Here's how the part is built. I have some questions about the finished solid (model axes, mm). A direction names the side the tool comes from. Round coordinates to 2 decimals unless told otherwise and drop trailing zeros. Write each loop counter-clockwise with the first axis right and the second up, starting at its lowest first coordinate (ties: lowest second). Pieces come first, ordered by that corner, then holes. Notation, with made-up numbers: (1.25, 41) -> (18.25, 41) arc R30 ccw to (18.25, 78) -> close; hole circle Ø10 at (-6.75, -20). An arc over 180 degrees is marked (long way). Answer as CSV lines item,"result".
from build123d import *

# Parameters (mm, degrees)
CROQUIS1_W              = 75
CROQUIS1_H              = 75
SALIENTE_EXTRUIR1_DEPTH = 15
REDONDEO1_R             = 8
CROQUIS2_R              = 4
CORTAR_EXTRUIR1_DEPTH   = 15
SALIENTE_EXTRUIR2_DEPTH = 30
REDONDEO2_R             = 6
CROQUIS5_R              = 3
CORTAR_EXTRUIR2_DEPTH   = 54.5
CROQUIS6_R              = 5
CORTAR_EXTRUIR4_DEPTH   = 30
CROQUIS4_R              = 23
SALIENTE_EXTRUIR4_DEPTH = 5
CROQUIS8_R              = 12.5
CORTAR_EXTRUIR6_DEPTH   = 51


with BuildPart() as part:
    # Croquis1 → Saliente-Extruir1 (new body)
    with BuildSketch(Plane(origin=(0, 0, 0), x_dir=(1, 0, 0), z_dir=(0, 1, 0))):
        Rectangle(CROQUIS1_W, CROQUIS1_H)
    extrude(amount=SALIENTE_EXTRUIR1_DEPTH)

    # Redondeo1
    redondeo1_edges = [part.edges().sort_by_distance(p)[0] for p in [
        (37.5, 7.5, 37.5),
        (-37.5, 7.5, 37.5),
        (-37.5, 7.5, -37.5),
        (37.5, 7.5, -37.5),
    ]]
    fillet(redondeo1_edges, radius=REDONDEO1_R)

    # Croquis2 → Cortar-Extruir1 (cut)
    with BuildSketch(Plane(origin=(0, 15, 0), x_dir=(1, 0, 0), z_dir=(0, 1, 0))):
        with Locations((-29.5, 29.5)):
            Circle(CROQUIS2_R)
        with Locations((-29.5, -29.5)):
            Circle(CROQUIS2_R)
        with Locations((29.5, 29.5)):
            Circle(CROQUIS2_R)
        with Locations((29.5, -29.5)):
            Circle(CROQUIS2_R)
    extrude(amount=-CORTAR_EXTRUIR1_DEPTH, mode=Mode.SUBTRACT)

    # Croquis3 → Saliente-Extruir2 (add)
    with BuildSketch(Plane(origin=(0, 15, 0), x_dir=(1, 0, 0), z_dir=(0, 1, 0))):
        with BuildLine():
            Line((-16, -28.5), (-9, -28.5))
            Line((-9, -28.5), (-9, -17.5))
            Line((-9, -17.5), (9, -17.5))
            Line((9, -17.5), (9, -28.5))
            Line((9, -28.5), (16, -28.5))
            Line((16, -28.5), (16, -12.953381025))
            Line((16, -12.953381025), (27.733418669, -9.619169527))
            ThreePointArc((27.733418669, -9.619169527), (35, 0), (27.733418669, 9.619169527))
            Line((27.733418669, 9.619169527), (16, 12.953381025))
            Line((16, 12.953381025), (16, 28.5))
            Line((16, 28.5), (9, 28.5))
            Line((9, 28.5), (9, 17.5))
            Line((9, 17.5), (-9, 17.5))
            Line((-9, 17.5), (-9, 28.5))
            Line((-9, 28.5), (-16, 28.5))
            Line((-16, 28.5), (-16, 12.953381025))
            Line((-16, 12.953381025), (-27.733418669, 9.619169527))
            ThreePointArc((-27.733418669, 9.619169527), (-35, 0), (-27.733418669, -9.619169527))
            Line((-27.733418669, -9.619169527), (-16, -12.953381025))
            Line((-16, -12.953381025), (-16, -28.5))
        make_face()
    extrude(amount=SALIENTE_EXTRUIR2_DEPTH)

    # Redondeo2
    redondeo2_edges = [part.edges().sort_by_distance(p)[0] for p in [
        (-12.5, 45, 28.5),
        (12.5, 45, 28.5),
        (12.5, 45, -28.5),
        (-12.5, 45, -28.5),
    ]]
    fillet(redondeo2_edges, radius=REDONDEO2_R)

    # Croquis5 → Cortar-Extruir2 (cut, through all)
    with BuildSketch(Plane(origin=(16, 0, 0), x_dir=(0, 0, -1), z_dir=(1, 0, 0))):
        with Locations((-22.5, 39)):
            Circle(CROQUIS5_R)
        with Locations((22.5, 39)):
            Circle(CROQUIS5_R)
    extrude(amount=-CORTAR_EXTRUIR2_DEPTH, mode=Mode.SUBTRACT)

    # Croquis6 → Cortar-Extruir4 (cut)
    with BuildSketch(Plane(origin=(0, 45, 0), x_dir=(1, 0, 0), z_dir=(0, 1, 0))):
        with Locations((-25, 0)):
            Circle(CROQUIS6_R)
        with Locations((25, 0)):
            Circle(CROQUIS6_R)
    extrude(amount=-CORTAR_EXTRUIR4_DEPTH, mode=Mode.SUBTRACT)

    # Croquis4 → Saliente-Extruir4 (add)
    with BuildSketch(Plane(origin=(0, 0, 0), x_dir=(-1, 0, 0), z_dir=(0, -1, 0))):
        Circle(CROQUIS4_R)
    extrude(amount=SALIENTE_EXTRUIR4_DEPTH)

    # Croquis8 → Cortar-Extruir6 (cut, through all)
    with BuildSketch(Plane(origin=(0, 45, 0), x_dir=(1, 0, 0), z_dir=(0, 1, 0))):
        Circle(CROQUIS8_R)
    extrude(amount=-CORTAR_EXTRUIR6_DEPTH, mode=Mode.SUBTRACT)


solid = part.part
Item 1: Will these pins go through, and if not, where does the flat tip stop? pin 1 (3.5 mm diameter, centred on x = -13, y = 29, fed in from -Z); pin 2 (5 mm diameter, centred on x = 25.5, z = 1.5, fed in from +Y); pin 3 (13 mm diameter, centred on x = -29.5, z = 29.5, fed in from -Y); pin 4 (22.5 mm diameter, centred on x = 3.5, z = -4, fed in from +Y).
Results found:
pin 1,"stops at z = -28.5"
pin 2,"stops at y = 15"
pin 3,"stops at y = 0"
pin 4,"stops at y = 45"
Item 2: Suppose I cut it at B-B, the plane z = 2. List the corners of the cut face in (x, y) for me.
Results found:
outline,"(-37.5, 0) -> (-22.91, 0) -> (-22.91, -5) -> (-12.34, -5) -> (-12.34, 45) -> (-20.42, 45) -> (-20.42, 15) -> (-29.58, 15) -> (-29.58, 45) -> (-34.8, 45) -> (-34.8, 15) -> (-37.5, 15) -> close; (12.34, -5) -> (22.91, -5) -> (22.91, 0) -> (37.5, 0) -> (37.5, 15) -> (34.8, 15) -> (34.8, 45) -> (29.58, 45) -> (29.58, 15) -> (20.42, 15) -> (20.42, 45) -> (12.34, 45) -> close"
Item 3: Suppose I cut it at C-C, the plane x = 18. List the corners of the cut face in (y, z) for me.
Results found:
outline,"(-5, -14.32) -> (0, -14.32) -> (0, -37.5) -> (15, -37.5) -> (15, -12.39) -> (45, -12.39) -> (45, 12.39) -> (15, 12.39) -> (15, 37.5) -> (0, 37.5) -> (0, 14.32) -> (-5, 14.32) -> close"
Item 4: If we mould it in two halves opening along Z, with no side actions, what happens to faces 1 (the flat face through (9, 30, -23)), 2 (the flat face through (0, 7, 37.5)), 3 (the cylindrical face through (28.979, 7.605, -33.466))? For each: pulls with the +Z half, pulls with the -Z half, needs draft (parallel to the pull), parting line crosses it, or undercut.
Results found:
face 1,"needs draft"
face 2,"pulls with the +Z half"
face 3,"undercut"
Item 5: I need wall thicknesses on L1, parallel to X at y = 34.5, z = 0; L2, parallel to X at y = 12.25, z = -29.5. Which ranges of each line are inside material? Lowest first, please.
Results found:
L1,"x = -35 to -30, -20 to -12.5, 12.5 to 20, 30 to 35"
L2,"x = -37.5 to -33.5, -25.5 to 25.5, 33.5 to 37.5"
Item 6: For faces 4 (the cylindrical face through (35, 30, 0)), 5 (the flat face through (-16, 30, 21)), 6 (the flat face through (25, 15, 0)), 7 (the flat face through (12, 27, 28.5)), 8 (the flat face through (-9, 30, -23)), which set-ups out of +Z, -Z, +X, -X, +Y, -Y let a thin tool reach every point of the face, with its end or its side?
Results found:
face 4,"+X, +Y"
face 5,"+Z, -X, +Y"
face 6,"+Y"
face 7,"+Z, +X, -X, +Y"
face 8,"-Z, +Y"
Item 7: Suppose I cut it at A-A, the plane y = 20. List the corners of the cut face in (x, z) for me.
Results found:
outline,"(-27.73, -9.62) -> (-16, -12.95) -> (-16, -28.5) -> (-9, -28.5) -> (-9, -17.5) -> (9, -17.5) -> (9, -28.5) -> (16, -28.5) -> (16, -12.95) -> (27.73, -9.62) arc R10 ccw to (27.73, 9.62) -> (16, 12.95) -> (16, 28.5) -> (9, 28.5) -> (9, 17.5) -> (-9, 17.5) -> (-9, 28.5) -> (-16, 28.5) -> (-16, 12.95) -> (-27.73, 9.62) arc R10 ccw to start; hole circle Ø10 at (-25, 0); hole circle Ø25 at (0, 0); hole circle Ø10 at (25, 0)"
Item 8: Suppose I cut it at D-D, the plane x = -22. List the corners of the cut face in (y, z) for me.
Results found:
outline,"(-5, -6.71) -> (0, -6.71) -> (0, -37.5) -> (15, -37.5) -> (15, -11.25) -> (45, -11.25) -> (45, -4) -> (15, -4) -> (15, 4) -> (45, 4) -> (45, 11.25) -> (15, 11.25) -> (15, 37.5) -> (0, 37.5) -> (0, 6.71) -> (-5, 6.71) -> close"
